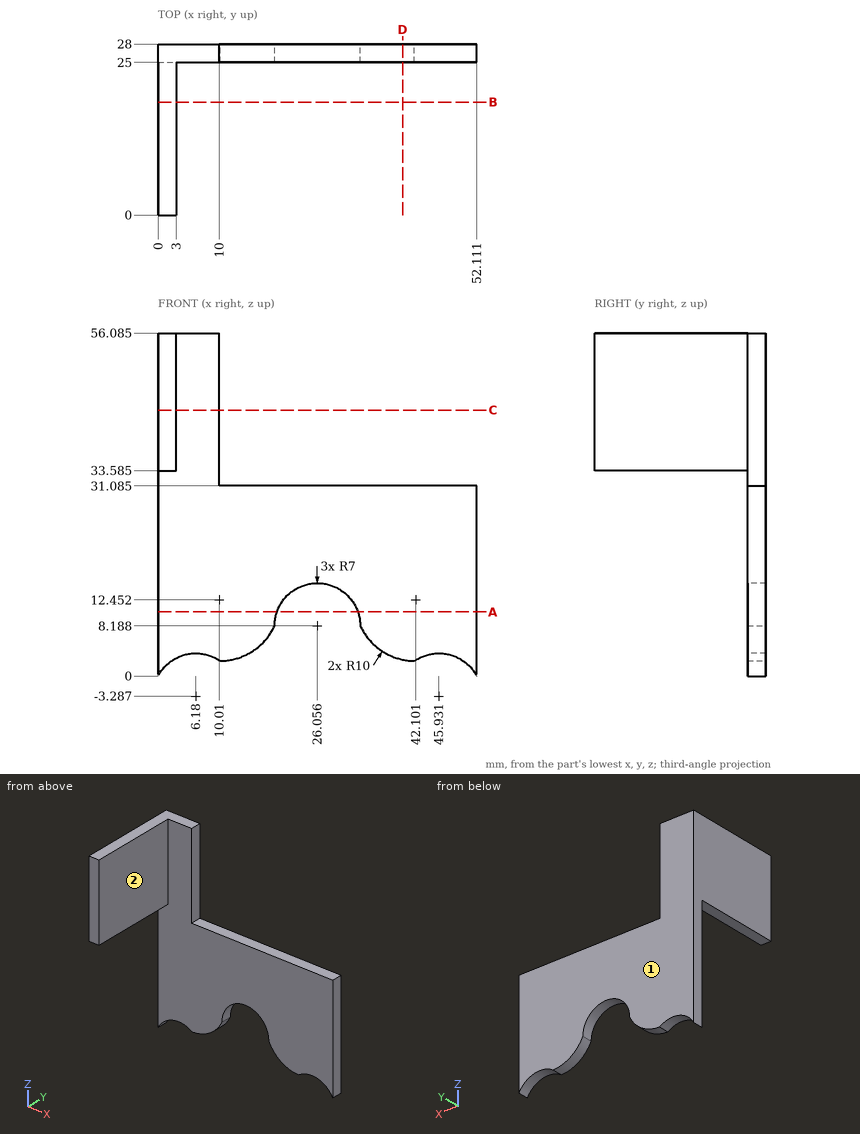
Geometry check sheet. Reference: drawing and pictorial views, mm from the part's lowest x, y, z. A direction names the side the tool comes from. Round coordinates to 2 decimals unless told otherwise and drop trailing zeros. Loops run counter-clockwise (first coordinate to the right, second up) from the corner with the lowest first, then second, coordinate; pieces in that order, holes last. Notation, with made-up numbers: M 48.25,52.5 L 97.25,52.5 A19 ccw 97.25,75.5 Z; hole C 36,-23.5 d4. An arc over 180 degrees is marked long. Return JSON: item names as keys, results as strings. Group by question number.
(1) Scan lines: line 1 along X through (y, z) = (26.25, 8.5); line 2 along X through (y, z) = (14.5, 52); line 3 along X through (y, z) = (25.25, 33.5). Record each from-to range of solid material in increasing order. Write a range as [from, to].
(2) Section check A-A, the plane z = 10.5. Enter the section's corners in (x, y), and give its area (3 significant figures).
(3) Section check D-D, the plane x = 40. Enter the section's corners in (y, z) (1 decimal).
(4) Section check C-C, the plane z = 43.5. Enter the section's corners in (x, y), and give its area (3 significant figures).
(5) Go/stop test with flat-tipped pins: pin 1 (0.9 mm diameter, centred on x = 22, y = 26.5, fed in from +Z) (3 decimals); pin 2 (8 mm diameter, centred on y = 19, z = 36, fed in from -X); pin 3 (1.5 mm diameter, centred on x = 1.5, y = 15, fed in from -Z) (3 decimals); pin 4 (15.5 mm diameter, centred on x = 26, z = 14.5, fed in from -Y). Record where each tip stops, or that it passes through.
(6) Set-up check for the marked faces 1 and 2: record each of +Z, -Z, +X, -X, +Y, -Y from which the full face is reachable in a straight line by a thin tool's end or side.
(7) Section check B-B, the plane y = 18.5. Enter the section's corners in (x, z) (1 decimal), and give its area (3 significant figures).
Data:
{
 "1": {"line 1": "[0, 19.06], [33.05, 52.11]", "line 2": "[0, 3]", "line 3": "[0, 10]"},
 "2": {"outline": "M 0,25 L 19.45,25 L 19.45,28 L 0,28 Z; M 32.66,25 L 52.11,25 L 52.11,28 L 32.66,28 Z", "area": "117 mm²"},
 "3": {"outline": "M 25,2.7 L 28,2.7 L 28,31.1 L 25,31.1 Z"},
 "4": {"outline": "M 0,0 L 3,0 L 3,25 L 10,25 L 10,28 L 0,28 Z", "area": "105 mm²"},
 "5": {"pin 1": "z = 31.085", "pin 2": "x = 0", "pin 3": "z = 33.585", "pin 4": "y = 25"},
 "6": {"face 1": "+Z, -Z, +X, -X, +Y", "face 2": "+Z, -Z, +X, -Y"},
 "7": {"outline": "M 0,33.6 L 3,33.6 L 3,56.1 L 0,56.1 Z", "area": "67.5 mm²"}
}
